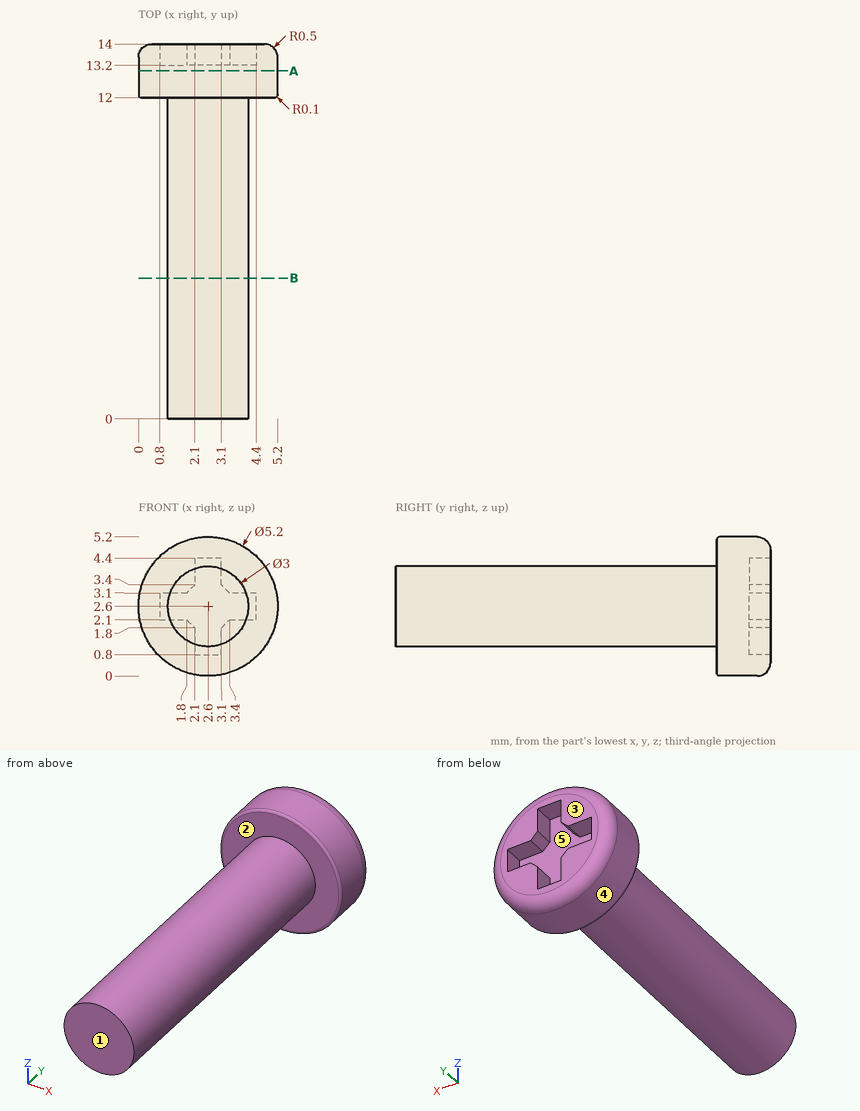
Input: dimensioned drawing with shaded views. Units: mm. Origin: part minimum x, y, z. A direction names the side the tool comes from. Coordinates: 2 decimals unless noted, no trailing zeros. Loops run counter-clockwise (first coordinate to the right, second up) from the corner with the lowest first, then second, coordinate; pieces in that order, holes last. Notation, with made-up numbers: M -23,84.5 L 3,84.5 A19 ccw 3,93.5 Z; hole C 62.5,30.25 d6. An arc over 180 degrees is marked long. Put each result on its own line as item: value.
(1) Cut plane B-B on y = 5.25. Return the cut outline in (x, z).
Answer sheet:
outline: C 2.6,2.6 d3
(2) Draft query along Z for the marked faces 3, 4 and 5. Return one class per face: pulls with the +Z half, pulls with the -Z half, needs draft (parallel to the pull), parting line crosses it, or undercut.
Answer sheet:
face 3: needs draft
face 4: parting line crosses it
face 5: undercut
(3) Material intervals for probe 1 along Y at (x, z) = (3.6, 2.45); probe 2 along Y at (x, z) = (1.25, 3.35); probe 3 along Z at (x, y) = (2.6, 4.75), sorted ascending.
Answer sheet:
probe 1: y = 0 to 13.2
probe 2: y = 12 to 14
probe 3: z = 1.1 to 4.1
(4) Cut plane A-A on y = 13. Return the cut outline in (x, z), then the cut area to 3 significant figures.
Answer sheet:
outline: C 2.6,2.6 d5.2
area: 21.2 mm^2
(5) Access query for the marked faces 1 and 2. Directions: +Z, -Z, +X, -X, +Y, -Y. A direction counts if a zero-diameter tool reaches every point of the face in a straight line with its end or side. Return the directions, or none.
Answer sheet:
face 1: +Z, -Z, +X, -X, -Y
face 2: -Y
(6) First-contact query: pin 1 (0.9 mm diameter, centred on x = 4, y = 13.5, fed in from +Z); pin 2 (0.6 mm diameter, centred on x = 1.5, y = 13.5, fed in from +Z); pin 3 (0.9 mm diameter, centred on y = 13.5, z = 4, fed in from -X). Flat tips, straight axial feed; report the tip coordinate or a pass-through.
Answer sheet:
pin 1: stops at z = 5.02
pin 2: stops at z = 5.07
pin 3: stops at x = 0.18
